Input: dimensioned drawing with shaded views. Units: mm. Origin: part minimum x, y, z. A direction names the side the tool comes from. Round coordinates to 2 decimals unless told otherwise and drop trailing zeros. Loops run counter-clockwise (first coordinate to the right, second up) from the corner with the lowest first, then second, coordinate; pieces in that order, holes last.
Item 1: Access query for the marked faces 1, 2 and 3. Directions: +Z, -Z, +X, -X, +Y, -Y. A direction counts if a zero-diameter tool reaches every point of the face in a straight line with its end or side. Return the directions, or none.
Item 2: Section query D-D on x = 4.75. Return loops of the section in (y, z) (3 decimals).
Item 3: Pull-direction query (Y, two-part tool) for the marked faces 4, 5 and 6; classes: released by +Y, released by -Y, zero draft, split by the parting line, or undercut.
Item 4: Ray query, L1, parallel to Y at x = 12.5, z = 20 (3 decimals); L2, parallel to Z at x = 0.75, y = 24; L3, parallel to X at y = 7, z = 10.5. Return the intervals inside material, ascending.
Item 5: First-contact query: P1, Ø8, axis at y = 6.5, z = 15, coming from the -X side; P2, Ø2, axis at y = 21, z = 14, coming from the +X side; P3, Ø5, axis at x = 8.5, y = 34.5, coming from the +Z side; P4, Ø8, axis at x = 11, y = 6.5, coming from the -Z side. Flat tips, straight axial feed; report the tip coordinate or a pass-through.
Item 6: Section query C-C on x = 1.5. Return loops of the section in (y, z) (3 decimals).
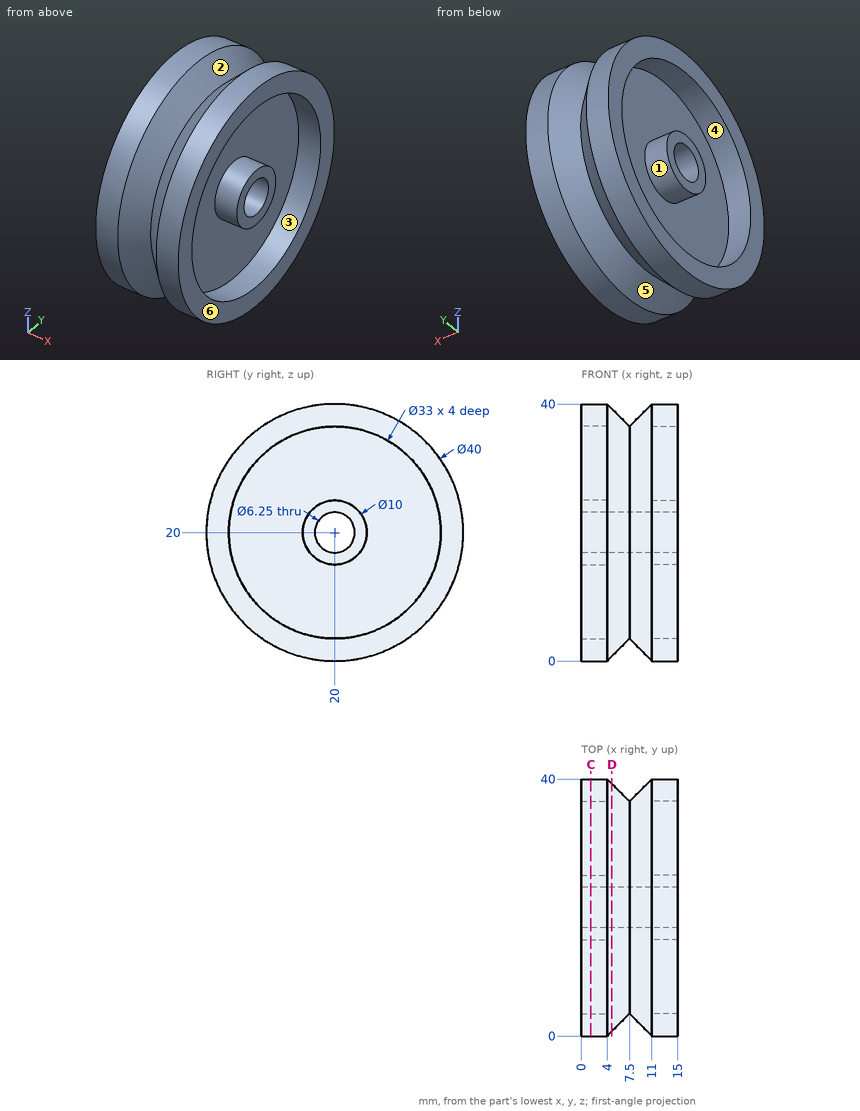
Data:
1. face 1: -X
1. face 2: none
1. face 3: +X
2. outline: circle Ø38.5 at (20, 20); hole circle Ø6.25 at (20, 20)
3. face 4: undercut
3. face 5: split by the parting line
3. face 6: zero draft
4. L1: y = 0 to 3.5, 15 to 16.875, 23.125 to 25, 36.5 to 40
4. L2: z = 0.4 to 3.99, 17 to 23, 36.01 to 39.6
4. L3: x = 4 to 11
5. P1: stops at x = 0
5. P2: stops at x = 11
5. P3: stops at z = 34.54
5. P4: stops at z = 2.4
6. outline: circle Ø40 at (20, 20); circle Ø10 at (20, 20); hole circle Ø33 at (20, 20); hole circle Ø6.25 at (20, 20)
